For this review, take the finished solid that the model builds, in its own axes (mm). A direction names the side the tool comes from. Round coordinates to 2 decimals unless told otherwise and drop trailing zeros. Order: outer loops, then holes, each group sorted by start corner. A loop starts at its lowest first (then second) coordinate and runs counter-clockwise, first axis right, second up. Notation, with made-up numbers: (-34.5, 55) - (8.5, 55) arc R22 cw to (8.5, 69) - close; hole circle Ø7 at (80.25, 71). An arc over 180 degrees is marked (long way). One line per item, written item: value.
```python
from build123d import *

# Parameters (mm, degrees)
F0_R     = 1.55
F0_W     = 30
F0_H     = 3
F1_DEPTH = 3
F2_W     = 30
F2_H     = 3
F3_DEPTH = 5
F4_R     = 1.55
F5_DEPTH = 3
F6_R     = 3
F7_F1_R  = 5
F7_F2_R  = 5
F7_F3_R  = 5
F7_F4_R  = 5
F7_F5_R  = 5
F7_F6_R  = 5


with BuildPart() as f1:
    # F0 (on Right) → F1 (new body)
    with BuildSketch(Plane.YZ):
        Polygon((-15, 4), (-25, 4), (-25, -4), (-15, -4), (-5, -1.5), (-5, 1.5), align=None)
        with Locations((-21, 0)):
            Circle(F0_R, mode=Mode.SUBTRACT)
        with Locations((10, 0)):
            Rectangle(F0_W, F0_H)
    extrude(amount=F1_DEPTH)

    # F2 (on face) → F3 (join)
    with BuildSketch(Plane.YZ.offset(3)):
        with Locations((10, 0)):
            Rectangle(F2_W, F2_H)
    extrude(amount=F3_DEPTH)

    # F4 (on face) → F5 (cut, through all)
    with BuildSketch(Plane(origin=(0, 0, -1.5), x_dir=(1, 0, 0), z_dir=(0, 0, -1))):
        Polygon((8, 5), (3, 5), (8, -5), align=None)
        with Locations((4, -21)):
            Circle(F4_R)
    extrude(amount=-F5_DEPTH, mode=Mode.SUBTRACT)

    # F6
    f6_edges = [f1.edges().sort_by_distance(p)[0] for p in [
        (1.5, -25, 4),
        (1.5, -25, -4),
        (8, 25, 0),
    ]]
    fillet(f6_edges, radius=F6_R)

    # F7: fillet of radius 5 on 6 edges, made by hand

    # F7_f1
    f7_f1_edges = [f1.edges().sort_by_distance(p)[0] for p in [
        (1.5, -15, 4),
    ]]
    fillet(f7_f1_edges, radius=F7_F1_R)

    # F7_f2
    f7_f2_edges = [f1.edges().sort_by_distance(p)[0] for p in [
        (1.5, -5, 1.5),
    ]]
    fillet(f7_f2_edges, radius=F7_F2_R)

    # F7_f3
    f7_f3_edges = [f1.edges().sort_by_distance(p)[0] for p in [
        (3, -5, 0.019016066),
    ]]
    fillet(f7_f3_edges, radius=F7_F3_R)

    # F7_f4
    f7_f4_edges = [f1.edges().sort_by_distance(p)[0] for p in [
        (1.5, -15, -4),
    ]]
    fillet(f7_f4_edges, radius=F7_F4_R)

    # F7_f5
    f7_f5_edges = [f1.edges().sort_by_distance(p)[0] for p in [
        (1.5706586412, -5, -1.5),
    ]]
    fillet(f7_f5_edges, radius=F7_F5_R)

    # F7_f6
    f7_f6_edges = [f1.edges().sort_by_distance(p)[0] for p in [
        (8, 5, 0),
    ]]
    fillet(f7_f6_edges, radius=F7_F6_R)


solid = f1.part
```
Item 1: Take a section at D-D (y = -2.5). Write out the cut boundary in (x, z), plus the area to 4 significant figures.
Returned:
outline: (0, -1.5) - (4.25, -1.5) - (4.25, 1.5) - (0, 1.5) - close
area: 12.75 mm^2
Item 2: Machinability: for faces 1 (the flat face through (4, 10, 1.5)), 2 (the flat face through (4, 10, -1.5)), 3 (the cylindrical face through (3.13, -5.05, 0.03)), which of the approach directions +Z, -Z, +X, -X, +Y, -Y give a long, thin tool a straight path to every point of the face, cutting with its end or side? Answer none if there is none.
Returned:
face 1: +Z, +X, -X, +Y
face 2: -Z, +X, -X, +Y
face 3: +Z, -Z, +X, -Y
Item 3: Take a section at B-B (x = 4). Write out the cut boundary in (y, z).
Returned:
outline: (-3, -1.5) - (19.45, -1.5) - (19.45, 1.5) - (-3, 1.5) - close; (22.55, -1.5) - (25, -1.5) - (25, 1.5) - (22.55, 1.5) - close
Item 4: Wall thickness on line 1 (X direction, y = 21, z = -0.55); line 2 (Z direction, x = 0.8, y = -21); line 3 (X direction, y = -21.5, z = 3): over which ranges is each line inside the solid? List them lowest first.
Returned:
line 1: 0 to 2.45, 5.55 to 8
line 2: -4 to -1.55, 1.55 to 4
line 3: 0 to 3
Item 5: The part is to be moulded in two halves that separate along Y. For faces 4 (the cylindrical face through (7.862, 5.016, 0.021)), 5 (the flat face through (0, -6, 0)), 6 (the cylindrical face through (3.798, 19.463, -0.021)), say which applies: +Y half, -Y half, draft (parallel to the pull), parting line (faces both ways), or undercut.
Returned:
face 4: -Y half
face 5: draft
face 6: undercut
Item 6: Take a section at A-A (z = 0). Write out the cut boundary in (x, y), plus the area to 3 significant figures.
Returned:
outline: (0, -25) - (3, -25) - (3, -22.55) - (0, -22.55) - close; (0, -19.45) - (3, -19.45) - (3, -6.18) arc R5 cw to (3.53, -3.94) - (7.47, 3.94) arc R5 ccw to (8, 6.18) - (8, 22) arc R3 ccw to (5, 25) - (0, 25) - close; hole circle Ø3.1 at (4, 21)
area: 256 mm^2
Item 7: For P1, Ø2.5, axis at y = -17.5, z = 1.5, coming from the +X side, flat-tipped, find the tip position at first contact; note if it passes through.
Returned:
P1: x = 3
Item 8: Take a section at C-C (y = 21). Write out the cut boundary in (x, z), plus the area to 3 significant figures.
Returned:
outline: (0, -1.5) - (2.45, -1.5) - (2.45, 1.5) - (0, 1.5) - close; (5.55, -1.5) - (8, -1.5) - (8, 1.5) - (5.55, 1.5) - close
area: 14.7 mm^2
